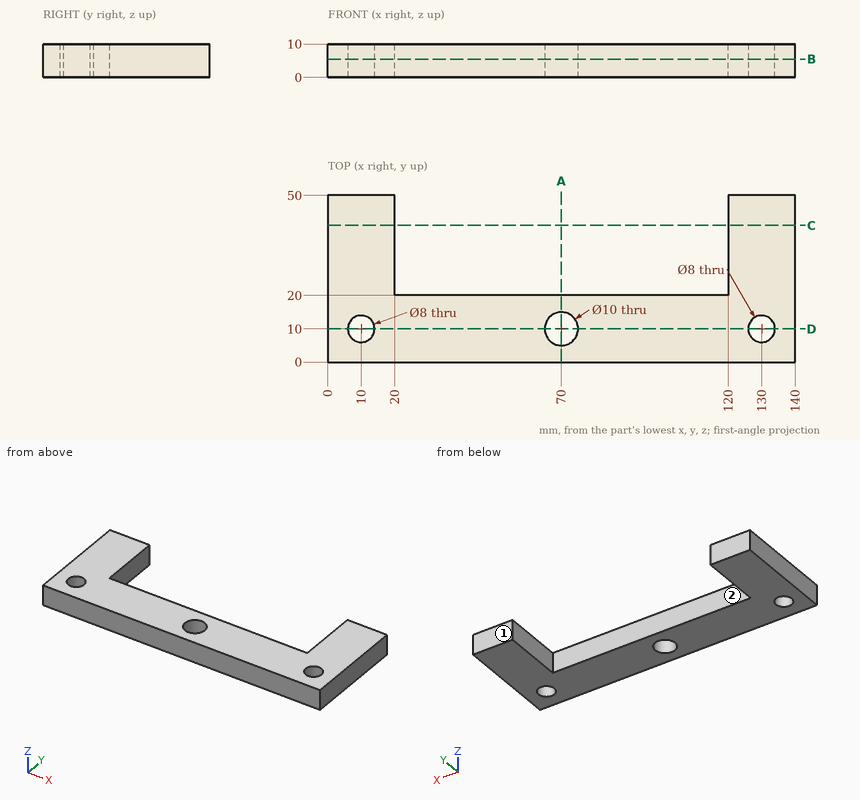
Verification items for this drawing (mm, ordinates from the low corner). A direction names the side the tool comes from. Round coordinates to 2 decimals unless told otherwise and drop trailing zeros. Loops run counter-clockwise (first coordinate to the right, second up) from the corner with the lowest first, then second, coordinate; pieces in that order, holes last. Notation, with made-up numbers: (88, -1) - (99, -1) arc R17 ccw to (99, 12) - close; hole circle Ø8 at (-9, -32.75). An arc over 180 degrees is marked (long way). Answer as CSV lines item,"result". Start each with the question number.
Item 1: Section check B-B (z = 5.5). Record the boundary of the cut face in (x, y), and give its area (3 significant figures).
Item 2: Set-up check for the marked faces 1 and 2: record each of +Z, -Z, +X, -X, +Y, -Y from which the full face is reachable in a straight line by a thin tool's end or side.
Item 3: Section check D-D (y = 10). Record the boundary of the cut face in (x, z).
Item 4: Depth check by flat-ended pin: P1, Ø3, axis at x = 86.5, z = 7, coming from the +Y side; P2, Ø6.5, axis at x = 10, y = 10, coming from the -Z side; P3, Ø11.5, axis at x = 70, y = 10, coming from the +Z side. Enter the tip coordinate at first touch or a pass-through.
Item 5: Section check C-C (y = 41). Record the boundary of the cut face in (x, z), and give its area (3 significant figures).
Item 6: Scan lines: line 1 (X direction, y = 23, z = 1); line 2 (Y direction, x = 70, z = 7.25); line 3 (Y direction, x = 130, z = 4.5). Record each from-to range of solid material in increasing order. Write a range as [from, to].
Item 7: Section check A-A (x = 70). Record the boundary of the cut face in (y, z).
Report:
1,outline,"(0, 0) - (140, 0) - (140, 50) - (120, 50) - (120, 20) - (20, 20) - (20, 50) - (0, 50) - close; hole circle Ø8 at (10, 10); hole circle Ø10 at (70, 10); hole circle Ø8 at (130, 10)"
1,area,"3,820 mm2"
2,face 1,"+Z, -Z, +X, -X, +Y"
2,face 2,"+Z, -Z, +Y"
3,outline,"(0, 0) - (6, 0) - (6, 10) - (0, 10) - close; (14, 0) - (65, 0) - (65, 10) - (14, 10) - close; (75, 0) - (126, 0) - (126, 10) - (75, 10) - close; (134, 0) - (140, 0) - (140, 10) - (134, 10) - close"
4,P1,"stops at y = 20"
4,P2,"passes through"
4,P3,"stops at z = 10"
5,outline,"(0, 0) - (20, 0) - (20, 10) - (0, 10) - close; (120, 0) - (140, 0) - (140, 10) - (120, 10) - close"
5,area,"400 mm2"
6,line 1,"x = [0, 20], [120, 140]"
6,line 2,"y = [0, 5], [15, 20]"
6,line 3,"y = [0, 6], [14, 50]"
7,outline,"(0, 0) - (5, 0) - (5, 10) - (0, 10) - close; (15, 0) - (20, 0) - (20, 10) - (15, 10) - close"
